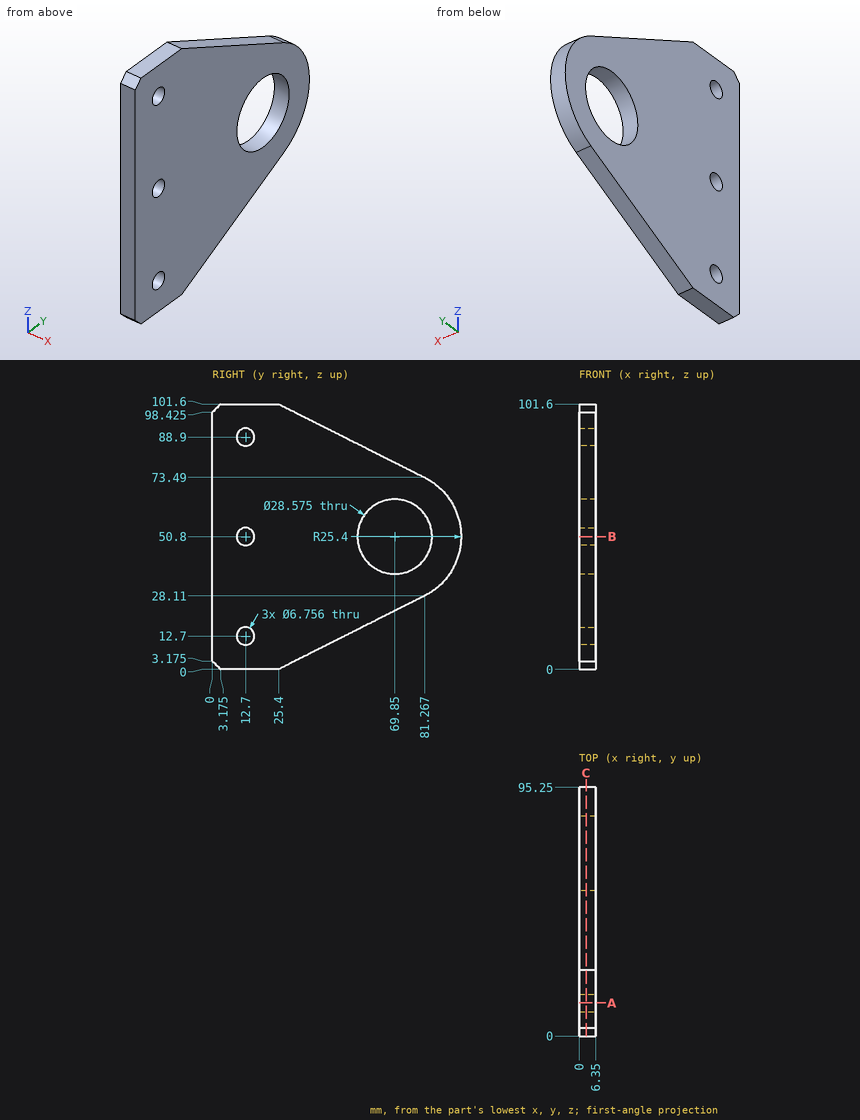
Can you work these out from the drawing? Everything is in mm from the part's minimum corner. Round coordinates to 2 decimals unless told otherwise and drop trailing zeros. Order: outer loops, then holes, each group sorted by start corner. A loop starts at its lowest first (then second) coordinate and runs counter-clockwise, first axis right, second up. Notation, with made-up numbers: (34.25, -4) - (91.25, -4) arc R28 cw to (91.25, 23) - close; hole circle Ø1 at (11.25, 0). An arc over 180 degrees is marked (long way). Answer in a Markdown table with one row per item.
(1) Please list where these lines run through material, in increasing order: L1, parallel to Y at x = 1.5, z = 50.8; L2, parallel to Y at x = 0.5, z = 49 (1 decimal); L3, parallel to Y at x = 4.25, z = 56. Write a range as from..to.
From the geometry:
| item | result |
|---|---|
| L1 | y = 0..9.32, 16.08..55.56, 84.14..95.25 |
| L2 | y = 0..9.8, 15.6..55.7, 84..95.2 |
| L3 | y = 0..56.54, 83.16..94.71 |
(2) Suppose I cut it at B-B, the plane z = 50.8. Please give me the cut outline in (x, y).
From the geometry:
| item | result |
|---|---|
| outline | (0, 0) - (6.35, 0) - (6.35, 9.32) - (0, 9.32) - close; (0, 16.08) - (6.35, 16.08) - (6.35, 55.56) - (0, 55.56) - close; (0, 84.14) - (6.35, 84.14) - (6.35, 95.25) - (0, 95.25) - close |
(3) Suppose I cut it at C-C, the plane x = 2.75. Count the separate pieces of the cut face and the enclosed holes in it, plus the area to 3 significant figures.
From the geometry:
| item | result |
|---|---|
| separate pieces | 1 |
| enclosed holes | 4 |
| area | 6,380 mm2 |
(4) Suppose I cut it at A-A, the plane y = 12.7. Please give me the cut outline in (x, z).
From the geometry:
| item | result |
|---|---|
| outline | (0, 0) - (6.35, 0) - (6.35, 9.32) - (0, 9.32) - close; (0, 16.08) - (6.35, 16.08) - (6.35, 47.42) - (0, 47.42) - close; (0, 54.18) - (6.35, 54.18) - (6.35, 85.52) - (0, 85.52) - close; (0, 92.28) - (6.35, 92.28) - (6.35, 101.6) - (0, 101.6) - close |
